Design review of the part built by this model. Coordinates are the model's own, in mm. Face numbers are marked on the shaded views. A direction names the side the tool comes from. Coordinates: 2 decimals unless noted, no trailing zeros. Loops run counter-clockwise (first coordinate to the right, second up) from the corner with the lowest first, then second, coordinate; pieces in that order, holes last. Notation, with made-up numbers: (33, 11.5) - (50, 11.5) arc R37 ccw to (50, 50.5) - close; hole circle Ø7 at (7.25, 0.5). An arc over 180 degrees is marked (long way). Use one line per item in the form item = value. Start each with the question number.
(1) The part is to be moulded in two halves that separate along X. For the marked faces 4, 5 and 6, say which applies: pulls with the +X half, pulls with the -X half, needs draft (parallel to the pull), parting line crosses it, or undercut.
(2) Add section B-B (y = -84). State the section outline as (x, z) points, plus the area to 3 significant figures.
(3) Tool access review of the marked faces 1, 2 and 3: name each direction out of +Z, -Z, +X, -X, +Y, -Y from which nothing blocks a thin tool from reaching the whole face with its end or side.
(4) Clearance check with flat-ended pins moving along their axes: pin 1 Ø1 at (x, y) = (-173, -79.5) entering from -Z; pin 2 Ø3 at (x, z) = (-157, 174) entering from -Y (3 decimals); pin 3 Ø4 at (x, y) = (-157.1, -80.5) entering from +Z. State where each tip first meets the part, or that it passes through.
(5) Add section D-D (x = -174). State the section outline as (y, z) points, plus the area to 3 significant figures.
(6) Add section C-C (z = 177.5). State the section outline as (x, y) points.
(7) Add section A-A (x = -166.1). State the section outline as (y, z) points, plus the area to 3 significant figures.
(8) For L1, parallel to X at y = -80.5, z = 176.5; L2, parallel to Y at x = -157.1, z = 178.05; L3, parallel to Y at x = -166.1, z = 178, list the stretches that pass through material, from the lowest coordinate up.
```python
from build123d import *

# Parameters (mm, degrees)
BOSS_EXTRUDE1_DEPTH          = 3.5
SKETCH2_W                    = 5
SKETCH2_H                    = 2
SKETCH3_W                    = 5.1
SKETCH3_H                    = 5
F_3_0_3_DIAMETER_HOLE1_D     = 3
F_3_0_3_DIAMETER_HOLE1_DEPTH = 8.5
F_8_0_8_DIAMETER_HOLE1_D     = 8
F_8_0_8_DIAMETER_HOLE1_DEPTH = 10.5


with BuildPart() as part:
    # Sketch1 → Boss-Extrude1 (new body)
    with BuildSketch(Plane(origin=(0, 0, 177.026431985), x_dir=(-1, 0, 0), z_dir=(0, 0, -1))):
        with BuildLine():
            Line((177.813226718, -74.200057886), (154.386773282, -74.200057886))
            ThreePointArc((154.386773282, -74.200057886), (152.6, -80.500057886), (154.386773282, -86.800057886))
            Line((154.386773282, -86.800057886), (177.813226718, -86.800057886))
            ThreePointArc((177.813226718, -86.800057886), (179.6, -80.500057886), (177.813226718, -74.200057886))
        make_face()
    extrude(amount=-BOSS_EXTRUDE1_DEPTH)

    # Sketch2 → Revolve1 (revolve)
    with BuildSketch(Plane(origin=(0, -80.500057886, 0), x_dir=(1, 0, 0), z_dir=(0, 1, 0))):
        with Locations((-163.6, -181.526431985)):
            Rectangle(SKETCH2_W, SKETCH2_H)
    revolve(axis=Axis((-166.1, -80.500057886, 180.526431985), (0, 0, 1)))

    # Sketch3 → Revolve2 (revolve)
    with BuildSketch(Plane.XZ.offset(80.500057886)):
        with Locations((-163.55, 174.526431985)):
            Rectangle(SKETCH3_W, SKETCH3_H)
    revolve(axis=Axis((-166.1, -80.500057886, 177.026431985), (0, 0, -1)))

    # Ø3.0 (3) Diameter Hole1
    with Locations(Plane.XY.offset(180.526431985)):
        with Locations((-157.1, -80.500057886), (-175.1, -80.500057886)):
            Hole(F_3_0_3_DIAMETER_HOLE1_D / 2, depth=F_3_0_3_DIAMETER_HOLE1_DEPTH)

    # Ø8.0 (8) Diameter Hole1
    with Locations(Plane(origin=(0, 0, 172.026431985), x_dir=(-1, 0, 0), z_dir=(0, 0, -1))):
        with Locations((166.1, -80.500057886)):
            Hole(F_8_0_8_DIAMETER_HOLE1_D / 2, depth=F_8_0_8_DIAMETER_HOLE1_DEPTH)


solid = part.part
```
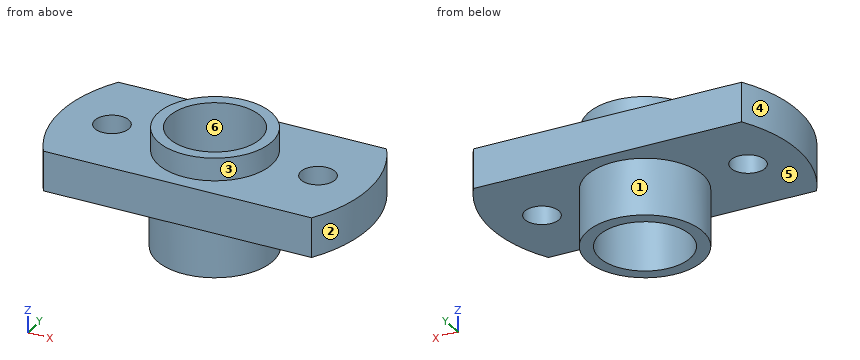
Computed values:
q1.face_4 = pulls with the -X half
q1.face_5 = needs draft
q1.face_6 = undercut
q2.outline = (-179.08, 177.03) - (-169.81, 177.03) - (-169.81, 172.03) - (-168.04, 172.03) - (-168.04, 182.53) - (-169.67, 182.53) - (-169.67, 180.53) - (-179.08, 180.53) - close; (-164.16, 172.03) - (-162.39, 172.03) - (-162.39, 177.03) - (-153.12, 177.03) - (-153.12, 180.53) - (-162.53, 180.53) - (-162.53, 182.53) - (-164.16, 182.53) - close
q2.area = 102 mm^2
q3.face_1 = -Z
q3.face_2 = +Z, -Z, +X
q3.face_3 = +Z
q4.pin_1 = 177.03
q4.pin_2 = through
q4.pin_3 = 180.53
q5.outline = (-86.8, 177.03) - (-81.52, 177.03) - (-81.52, 180.53) - (-86.8, 180.53) - close; (-79.48, 177.03) - (-74.2, 177.03) - (-74.2, 180.53) - (-79.48, 180.53) - close
q5.area = 37.0 mm^2
q6.outline = (-177.81, -86.8) - (-154.39, -86.8) arc R12 ccw to (-154.39, -74.2) - (-177.81, -74.2) arc R12 ccw to start; hole circle Ø3 at (-175.1, -80.5); hole circle Ø8 at (-166.1, -80.5); hole circle Ø3 at (-157.1, -80.5)
q7.outline = (-86.8, 177.03) - (-85.6, 177.03) - (-85.6, 172.03) - (-84.5, 172.03) - (-84.5, 182.53) - (-85.5, 182.53) - (-85.5, 180.53) - (-86.8, 180.53) - close; (-76.5, 172.03) - (-75.4, 172.03) - (-75.4, 177.03) - (-74.2, 177.03) - (-74.2, 180.53) - (-75.5, 180.53) - (-75.5, 182.53) - (-76.5, 182.53) - close
q7.area = 31.1 mm^2
q8.L1 = -171.2 to -170.1, -162.1 to -161
q8.L2 = -86.8 to -82, -79 to -74.2
q8.L3 = -86.8 to -84.5, -76.5 to -74.2
